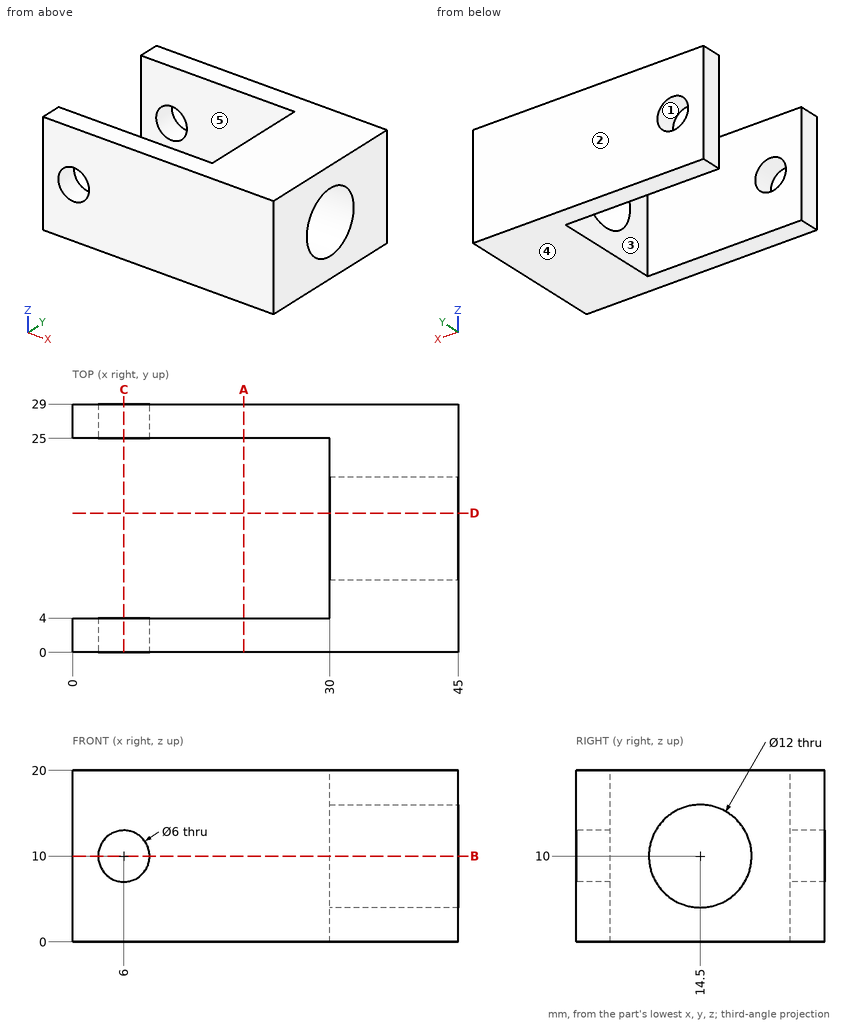
Design review of the part shown in the three views and the two pictorial views. Dimensions are in mm from the part's minimum x, y and z. A direction names the side the tool comes from. Coordinates: 2 decimals unless noted, no trailing zeros. Write each loop counter-clockwise with the first axis right and the second up, starting at its lowest first coordinate (ties: lowest second). Pieces come first, ordered by that corner, then holes.
(1) Tool access review of the marked faces 4 and 5: name each direction out of +Z, -Z, +X, -X, +Y, -Y from which nothing blocks a thin tool from reaching the whole face with its end or side.
(2) The part is to be moulded in two halves that separate along Y. For the marked faces 1, 2 and 3, say which applies: +Y half, -Y half, draft (parallel to the pull), parting line (faces both ways), or undercut.
(3) Add section D-D on y = 16.25. Give the boundary of the cut face in (x, z).
(4) Add section A-A on x = 20. Give the boundary of the cut face in (y, z), then the cut area to 3 significant figures.
(5) For pin 1 Ø5 at (x, y) = (6.5, 4) entering from -Z; pin 2 Ø3 at (y, z) = (16.5, 5.5) entering from -X, all flat-tipped, find the tip position at first contact; note any pin that passes through.
(6) Add section C-C on x = 6. Give the boundary of the cut face in (y, z).
(7) Add section B-B on z = 10. Give the boundary of the cut face in (x, y).
(8) Wall thickness on probe 1 along Z at (x, y) = (6, 0.95); probe 2 along Y at (x, z) = (41, 10); probe 3 along Y at (x, z) = (24, 16.5): over which ranges is each line inside the solid? List them lowest first.
Answer sheet:
1. face 4: -Z, +X, -X, +Y, -Y
1. face 5: +Z, -Z, -X
2. face 1: draft
2. face 2: +Y half
2. face 3: undercut
3. outline: (30, 0) - (45, 0) - (45, 4.26) - (30, 4.26) - close; (30, 15.74) - (45, 15.74) - (45, 20) - (30, 20) - close
4. outline: (0, 0) - (4, 0) - (4, 20) - (0, 20) - close; (25, 0) - (29, 0) - (29, 20) - (25, 20) - close
4. area: 160 mm2
5. pin 1: stops at z = 0
5. pin 2: stops at x = 30
6. outline: (0, 0) - (4, 0) - (4, 7) - (0, 7) - close; (0, 13) - (4, 13) - (4, 20) - (0, 20) - close; (25, 0) - (29, 0) - (29, 7) - (25, 7) - close; (25, 13) - (29, 13) - (29, 20) - (25, 20) - close
7. outline: (0, 0) - (3, 0) - (3, 4) - (0, 4) - close; (0, 25) - (3, 25) - (3, 29) - (0, 29) - close; (9, 0) - (45, 0) - (45, 8.5) - (30, 8.5) - (30, 4) - (9, 4) - close; (9, 25) - (30, 25) - (30, 20.5) - (45, 20.5) - (45, 29) - (9, 29) - close
8. probe 1: z = 0 to 7, 13 to 20
8. probe 2: y = 0 to 8.5, 20.5 to 29
8. probe 3: y = 0 to 4, 25 to 29
